The model under review builds one solid part; all positions refer to its coordinate system, in mm. A direction names the side the tool comes from. Coordinates: 2 decimals unless noted, no trailing zeros. Order: outer loops, then holes, each group sorted by start corner. A loop starts at its lowest first (then second) coordinate and runs counter-clockwise, first axis right, second up. Notation, with made-up numbers: M 45,-29 L 97,-29 A15 ccw 97,-19 Z; hole C -18.5,-18 d4. An arc over 180 degrees is marked long. One line per item, written item: value.
```python
from build123d import *

# Parameters (mm, degrees)
F1_DEPTH = 2
F2_R     = 1.19
F2_R_2   = 4.96
F3_DEPTH = 2.001


with BuildPart() as f1:
    # F0 (on Front) → F1 (new body)
    with BuildSketch(Plane.XZ):
        Polygon((65, 65), (0, 65), (-65, 65), (-65, -65), (0, -65), (65, -65), align=None)
    extrude(amount=-F1_DEPTH)

    # F2 (on Front) → F3 (cut, through all)
    with BuildSketch(Plane.XZ):
        with BuildLine():
            ThreePointArc((-3, 47.923168), (-4.080113, 50.311237), (-6.586714, 51.077052))
            ThreePointArc((-6.586714, 51.077052), (-36.415999, 36.415999), (-51.077052, 6.586714))
            ThreePointArc((-51.077052, 6.586714), (-50.311237, 4.080113), (-47.923168, 3))
            Line((-47.923168, 3), (-15.492902, 3))
            ThreePointArc((-15.492902, 3), (-13.708845, 3.547598), (-12.539219, 5.001799))
            ThreePointArc((-12.539219, 5.001799), (-9.545942, 9.545942), (-5.001799, 12.539219))
            ThreePointArc((-5.001799, 12.539219), (-3.547598, 13.708845), (-3, 15.492902))
            Line((-3, 15.492902), (-3, 47.923168))
        make_face()
        with BuildLine():
            ThreePointArc((6.586714, 51.077052), (4.080113, 50.311237), (3, 47.923168))
            Line((3, 47.923168), (3, 15.492902))
            ThreePointArc((3, 15.492902), (3.547598, 13.708845), (5.001799, 12.539219))
            ThreePointArc((5.001799, 12.539219), (9.545942, 9.545942), (12.539219, 5.001799))
            ThreePointArc((12.539219, 5.001799), (13.708845, 3.547598), (15.492902, 3))
            Line((15.492902, 3), (47.923168, 3))
            ThreePointArc((47.923168, 3), (50.311237, 4.080113), (51.077052, 6.586714))
            ThreePointArc((51.077052, 6.586714), (36.415999, 36.415999), (6.586714, 51.077052))
        make_face()
        with BuildLine():
            Line((-15.492902, -3), (-47.923168, -3))
            ThreePointArc((-47.923168, -3), (-50.311237, -4.080113), (-51.077052, -6.586714))
            ThreePointArc((-51.077052, -6.586714), (-36.415999, -36.415999), (-6.586714, -51.077052))
            ThreePointArc((-6.586714, -51.077052), (-4.080113, -50.311237), (-3, -47.923168))
            Line((-3, -47.923168), (-3, -15.492902))
            ThreePointArc((-3, -15.492902), (-3.547598, -13.708845), (-5.001799, -12.539219))
            ThreePointArc((-5.001799, -12.539219), (-9.545942, -9.545942), (-12.539219, -5.001799))
            ThreePointArc((-12.539219, -5.001799), (-13.708845, -3.547598), (-15.492902, -3))
        make_face()
        with BuildLine():
            ThreePointArc((5.001799, -12.539219), (3.547598, -13.708845), (3, -15.492902))
            Line((3, -15.492902), (3, -47.923168))
            ThreePointArc((3, -47.923168), (4.080113, -50.311237), (6.586714, -51.077052))
            ThreePointArc((6.586714, -51.077052), (36.415999, -36.415999), (51.077052, -6.586714))
            ThreePointArc((51.077052, -6.586714), (50.311237, -4.080113), (47.923168, -3))
            Line((47.923168, -3), (15.492902, -3))
            ThreePointArc((15.492902, -3), (13.708845, -3.547598), (12.539219, -5.001799))
            ThreePointArc((12.539219, -5.001799), (9.545942, -9.545942), (5.001799, -12.539219))
        make_face()
        with Locations((-8, 0)):
            Circle(F2_R)
        with Locations((8, 0)):
            Circle(F2_R)
        Circle(F2_R_2)
    extrude(amount=-F3_DEPTH, mode=Mode.SUBTRACT)


solid = f1.part
```
(1) Mouldability with a two-part tool opening along Z and no side actions: class faces 3 (the flat face through (-15, 0, 1)), 4 (the cylindrical face through (-4.052, 0.986, 50.286)) as +Z half, -Z half, draft (parallel to the pull), parting line (faces both ways), or undercut.
Geometry results:
face 3: draft
face 4: undercut
(2) We need section B-B, the plane x = 0. State the section outline as (y, z) points.
Geometry results:
outline: M 0,-65 L 2,-65 L 2,-4.96 L 0,-4.96 Z; M 0,4.96 L 2,4.96 L 2,65 L 0,65 Z
(3) For L1, parallel to Z at x = 0, y = 1.15; L2, parallel to Z at x = -42, y = 0.6; L3, parallel to X at y = 1.1, z = -21.5, list the stretches that pass through material, from the lowest coordinate up.
Geometry results:
L1: z = -65 to -4.96, 4.96 to 65
L2: z = -65 to -29.8, -3 to 3, 29.8 to 65
L3: x = -65 to -46.8, -3 to 3, 46.8 to 65
(4) Tool access review of faces 1 (the cylindrical face through (36.08, 0.99, -36.75)), 2 (the flat face through (-15, 2, 1)): name each direction out of +Z, -Z, +X, -X, +Y, -Y from which nothing blocks a thin tool from reaching the whole face with its end or side.
Geometry results:
face 1: +Y, -Y
face 2: +Z, -Z, +X, -X, +Y
(5) We need section A-A, the plane z = 43. State the section outline as (x, y) points.
Geometry results:
outline: M -65,0 L -28.34,0 L -28.34,2 L -65,2 Z; M -3,0 L 3,0 L 3,2 L -3,2 Z; M 28.34,0 L 65,0 L 65,2 L 28.34,2 Z
(6) We need section C-C, the plane y = 1. Count the separate pieces of the cut face and the enclosed holes in it, plus the area to 4 significant figures.
Geometry results:
separate pieces: 1
enclosed holes: 7
area: 10,000 mm2
(7) We need section D-D, the plane z = 28. State the section outline as (x, y) points, plus the area to 3 significant figures.
Geometry results:
outline: M -65,0 L -43.22,0 L -43.22,2 L -65,2 Z; M -3,0 L 3,0 L 3,2 L -3,2 Z; M 43.22,0 L 65,0 L 65,2 L 43.22,2 Z
area: 99.1 mm2
